Input: part model. Units: mm. Frame: model coordinates. Coordinates: 2 decimals unless noted, no trailing zeros. Order: outer loops, then holes, each group sorted by start corner. A loop starts at its lowest first (then second) coordinate and runs counter-clockwise, first axis right, second up. Notation, with made-up numbers: (24, 62.25) -> (59, 62.25) arc R5 cw to (59, 66.25) -> close; hole circle Ø11 at (-2, -28.75). An arc over 180 degrees is marked (long way). Use CSV: the item, a comma, the result in double quotes. Start each with the question number.
Autodesk Fusion 360 part; units mm, degrees
sketch "Skizze1" plane through (0, 0, 0) normal (0, 0, 1) x (1, 0, 0)
  line L0 (45, -30) -> (45, -50)
  line L1 (45, -50) -> (-45, -50)
  line L2 (-45, -50) -> (-45, -30)
  arc A0 (45, 0) -> (-45, 0) centre (0, 0) ccw
  line L3 (-45, 0) -> (-36, 0)
  line L4 (-36, 0) -> (-36, -30)
  line L5 (-36, -30) -> (-45, -30)
  line L6 (36, 0) -> (36, -30)
  line L7 (36, -30) -> (45, -30)
  line L8 (36, 0) -> (45, 0)
  dimension "d1" = 90
  dimension "d2" = 50
  dimension "d3" = 9
  dimension "d4" = 30
  dimension "d5" = 9
  dimension "d6" = 30
extrude "Extrusion1" add sketch "Skizze1" along normal blind 1.6
sketch "Skizze2" plane through (0, 0, 1.6) normal (0, 0, 1) x (-1, 0, 0)
  line L0 (-36, 30) -> (-36, 0)
  line L1 (-36, 0) -> (-45, 0)
  arc A0 (-45, 0) -> (45, 0) centre (0, 0) ccw
  line L2 (45, 0) -> (36, 0)
  line L3 (36, 0) -> (36, 30)
  line L4 (36, 30) -> (45, 30)
  line L5 (45, 30) -> (45, 50)
  line L6 (45, 50) -> (-45, 50)
  line L7 (-45, 50) -> (-45, 30)
  line L8 (-45, 30) -> (-36, 30)
  line L9 (36, 15) -> (36, 24)
  line L10 (36, 15) -> (36, 6)
  circle A1 centre (26, 24) radius 1.5
  circle A2 centre (16, 24) radius 1.5
  circle A3 centre (26, 6) radius 1.5
  circle A4 centre (16, 6) radius 1.5
  line L11 (36, 15) -> (36, 9)
  line L12 (36, 9) -> (11, 9)
  line L13 (11, 9) -> (11, 21)
  line L14 (11, 21) -> (36, 21)
  line L15 (36, 21) -> (36, 9)
  line L16 (36, 24) -> (36, 27)
  line L17 (36, 27) -> (4, 27)
  line L18 (4, 27) -> (4, 2)
  line L19 (4, 2) -> (36, 2)
  line L20 (36, 2) -> (36, 27)
  line L21 (4, 27) -> (-36, 27)
  line L22 (-36, 27) -> (-4, 27)
  line L23 (-4, 27) -> (-4, 2)
  line L24 (-4, 2) -> (-36, 2)
  line L25 (-36, 2) -> (-36, 27)
  line L26 (-11, 21) -> (-36, 21)
  line L27 (-36, 21) -> (-11, 21)
  line L28 (-11, 21) -> (-11, 9)
  line L29 (-11, 9) -> (-36, 9)
  line L30 (-36, 9) -> (-36, 21)
  circle A5 centre (-16, 6) radius 1.5
  circle A6 centre (-26, 6) radius 1.5
  circle A7 centre (-16, 24) radius 1.5
  circle A8 centre (-26, 24) radius 1.5
  dimension "d10" = 9
  dimension "d11" = 9
  dimension "d12" = 10
  dimension "d13" = 10
  dimension "d14" = 10
  dimension "d15" = 10
  dimension "d16" = 3
  dimension "d17" = 3
  dimension "d18" = 3
  dimension "d19" = 3
  dimension "d20" = 6
  dimension "d21" = 25
  dimension "d22" = 12
  dimension "d23" = 3
  dimension "d24" = 32
  dimension "d25" = 25
  dimension "d30" = 32
  dimension "d31" = 25
  dimension "d32" = 25
  dimension "d33" = 12
  dimension "d35" = 10
  dimension "d37" = 10
  dimension "d38" = 3
  dimension "d39" = 3
  dimension "d40" = 3
  dimension "d41" = 3
  dimension "d42" = 10
  dimension "d43" = 10
extrude "Extrusion2" cut sketch "Skizze2" against normal blind 1.6 contours A1 | A2 | A3 | A4
mirror "Spiegeln1" about plane through (0, 0, 0) normal (1, 0, 0) of "Extrusion2"
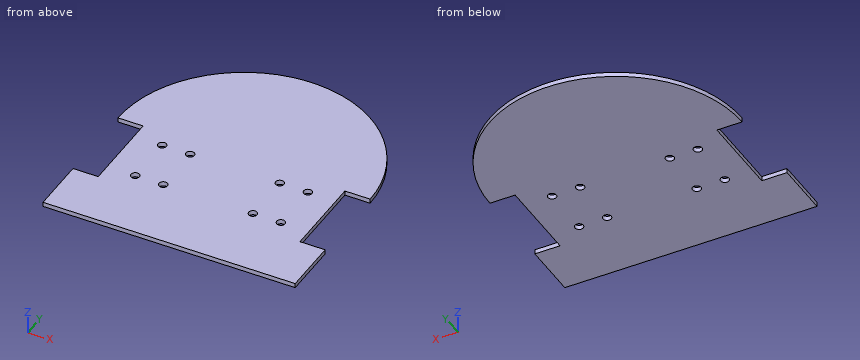
1. Section C-C on x = 16. Return loops of the section in (y, z), then the cut area to 3 significant figures.
2. Section A-A on y = -6. Return loops of the section in (x, z).
3. Section B-B on z = 0.3. State how many separate pieces and enclosed holes the cut face has, then the cut area to 3 significant figures.
4. Material intervals for line 1 along X through (y, z) = (-24, 1); line 2 along Y through (x, z) = (16, 1.15); line 3 along Y through (x, z) = (26, 1.05), sorted ascending.
5. Section D-D on x = 37.5. Return loops of the section in (y, z).
6. Contact query for flat-ended pins moving along their axis: P1, Ø0.5, axis at y = -18.5, z = 1, coming from the -X side; P2, Ø0.5, axis at y = -8.5, z = 1, coming from the +X side. Output: stop coordinate, or through.
Values follow:
1,outline,"(-50, 0) -> (-25.5, 0) -> (-25.5, 1.6) -> (-50, 1.6) -> close; (-22.5, 0) -> (-7.5, 0) -> (-7.5, 1.6) -> (-22.5, 1.6) -> close; (-4.5, 0) -> (42.06, 0) -> (42.06, 1.6) -> (-4.5, 1.6) -> close"
1,area,"138 mm2"
2,outline,"(-36, 0) -> (-27.5, 0) -> (-27.5, 1.6) -> (-36, 1.6) -> close; (-24.5, 0) -> (-17.5, 0) -> (-17.5, 1.6) -> (-24.5, 1.6) -> close; (-14.5, 0) -> (14.5, 0) -> (14.5, 1.6) -> (-14.5, 1.6) -> close; (17.5, 0) -> (24.5, 0) -> (24.5, 1.6) -> (17.5, 1.6) -> close; (27.5, 0) -> (36, 0) -> (36, 1.6) -> (27.5, 1.6) -> close"
3,separate pieces,"1"
3,enclosed holes,"8"
3,area,"7,080 mm2"
4,line 1,"x = -36 to -27.5, -24.5 to -17.5, -14.5 to 14.5, 17.5 to 24.5, 27.5 to 36"
4,line 2,"y = -50 to -25.5, -22.5 to -7.5, -4.5 to 42.06"
4,line 3,"y = -50 to -25.5, -22.5 to -7.5, -4.5 to 36.73"
5,outline,"(-50, 0) -> (-30, 0) -> (-30, 1.6) -> (-50, 1.6) -> close; (0, 0) -> (24.87, 0) -> (24.87, 1.6) -> (0, 1.6) -> close"
6,P1,"stops at x = -36"
6,P2,"stops at x = 36"
